from build123d import *

# Parameters (mm, degrees)
SKETCH_R           = 7.6
PAD_DEPTH          = 50
PAD001_DEPTH       = 1
POLARPATTERN_COUNT = 2
CHAMFER_ANGLE      = 15
CHAMFER_SIZE       = 1
SKETCH002_R        = 7.1
POCKET_DEPTH       = 50.001


with BuildPart() as part:
    # Sketch → Pad (new body)
    with BuildSketch(Plane.XY):
        Circle(SKETCH_R)
    extrude(amount=PAD_DEPTH)

    # Sketch001 (on DatumPlane) → Pad001 (join)
    with BuildSketch(Plane(origin=(7.5, 0, 0), x_dir=(-1, 0, 0), z_dir=(0, 1, 0))):
        with BuildLine():
            Line((0.5, 0.321717), (0.5, 41.435605))
            Line((-11.54404, 8.344877), (0.5, 41.435605))
            ThreePointArc((-11.54404, 8.344877), (-11.429864, 5.729814), (-9.5, 3.961419))
            Line((-9.5, 3.961419), (0.5, 0.321717))
        make_face()
    pad001 = extrude(amount=PAD001_DEPTH)

    # PolarPattern: Pad001 ×2 about axis
    polarpattern_axis = Axis((0, 0, 0), (0, 0, 1))
    for i in range(1, POLARPATTERN_COUNT):
        add(pad001.rotate(polarpattern_axis, i * 360 / POLARPATTERN_COUNT))

    # Chamfer
    chamfer_edges = [part.edges().sort_by_distance(p)[0] for p in [
        (-7.6, 0, 50),
    ]]
    chamfer_side = part.faces().sort_by_distance((-7.6, 0, 49.45575))[0]
    chamfer(chamfer_edges, length=CHAMFER_SIZE, angle=CHAMFER_ANGLE, reference=chamfer_side)

    # Sketch002 (on Face12 of Chamfer) → Pocket (cut, through all)
    with BuildSketch(Plane.XY.offset(50)):
        Circle(SKETCH002_R)
    extrude(amount=-POCKET_DEPTH, mode=Mode.SUBTRACT)


solid = part.part
Could you check a few things on this model? Use its own coordinates, in mm. A direction names the side the tool comes from. Give positions to 0.01 mm unless a question says otherwise; leave off trailing zeros. Order: outer loops, then holes, each group sorted by start corner. A loop starts at its lowest first (then second) coordinate and runs counter-clockwise, first axis right, second up. Notation, with made-up numbers: (23.25, -6) -> (40.25, -6) arc R20 ccw to (40.25, 2) -> close; hole circle Ø10 at (-35, 30.5). An arc over 180 degrees is marked (long way). Answer in a Markdown table with one row per item. Add a question column.
Item 1: Imagine slicing it at D-D (z = 43). List the corners of the cut face in (x, y) for me.
Item 2: Imagine slicing it at B-B (z = 23). List the corners of the cut face in (x, y) for me, and give its area (3 significant figures).
Item 3: Imagine slicing it at A-A (x = 0). List the corners of the cut face in (y, z) for me.
Item 4: We'd pull the mould along Y, two halves only. Please class faces 1 (the flat face through (-12, -1, 16)), 2 (the cylindrical face through (-0.92, 7.04, 25.35)), 3 (the flat face through (13.37, 0.49, 23.94)): pulls with the +Y half, pulls with the -Y half, needs draft (parallel to the pull), parting line crosses it, or undercut.
Item 5: Imagine slicing it at C-C (x = -8.5). List the corners of the cut face in (y, z) for me, and give its area (3 significant figures).
Item 6: For faces 4 (the flat face through (12, 1, 16)), 5 (the flat face through (-12, 0, 16)), 6 (the flat face through (-2, 7, 0)), 7 (the flat face through (12, 0, 16)), which set-ups out of +Z, -Z, +X, -X, +Y, -Y let a thin tool reach every point of the face, with its end or its side?
Item 7: I'm going to push flat-ended pins straight in: P1, Ø1, axis at y = 3.5, z = 6.5, coming from the -X side; P2, Ø6, axis at x = -13.5, z = 18, coming from the -Y side; P3, Ø2, axis at y = 0, z = 15.5, coming from the +X side. Where does each tip first touch, or does it pass through?
Item 8: Please list where these lines run through material, in increasing order: probe 1 along Y at (x, z) = (0, 14); probe 2 along X at (y, z) = (3.5, 34); probe 3 along X at (y, z) = (2.75, 16.5).
Result:
| question | item | result |
|---|---|---|
| 1 | outline | circle Ø15.2 at (0, 0); hole circle Ø14.2 at (0, 0) |
| 2 | outline | (-13.71, -1) -> (-7.53, -1) arc R7.6 ccw to (7.6, 0) -> (13.71, 0) -> (13.71, 1) -> (7.53, 1) arc R7.6 ccw to (-7.6, 0) -> (-13.71, 0) -> close; hole circle Ø14.2 at (0, 0) |
| 2 | area | 35.4 mm2 |
| 3 | outline | (-7.6, 0) -> (-7.1, 0) -> (-7.1, 50) -> (-7.33, 50) -> (-7.6, 49) -> close; (7.1, 0) -> (7.6, 0) -> (7.6, 49) -> (7.33, 50) -> (7.1, 50) -> close |
| 4 | face 1 | pulls with the -Y half |
| 4 | face 2 | undercut |
| 4 | face 3 | needs draft |
| 5 | outline | (-1, 0.87) -> (0, 0.87) -> (0, 37.31) -> (-1, 37.31) -> close |
| 5 | area | 36.4 mm2 |
| 6 | face 4 | +Z, -Z, +X, +Y |
| 6 | face 5 | +Z, -Z, -X, +Y |
| 6 | face 6 | -Z, +X, -X, +Y, -Y |
| 6 | face 7 | +Z, -Z, +X, -Y |
| 7 | P1 | x = -6.98 |
| 7 | P2 | y = -1 |
| 7 | P3 | x = 16.8 |
| 8 | probe 1 | -7.6 to -7.1, 7.1 to 7.6 |
| 8 | probe 2 | -6.75 to -6.18, 6.18 to 6.75 |
| 8 | probe 3 | -7.09 to -6.55, 6.55 to 7.09 |
